Read the model definition and answer for the solid it produces. Units are mm, in the model's axes. Face numbers are marked on the shaded views. A direction names the side the tool comes from. Give positions to 0.01 mm unless a question says otherwise; leave off trailing zeros. Order: outer loops, then holes, each group sorted by start corner. A loop starts at its lowest first (then second) coordinate and runs counter-clockwise, first axis right, second up.
Item 1: The mould has two halves that part along Y. Classify the marked faces 3, 4 and 5: +Y half, -Y half, draft (parallel to the pull), parting line (faces both ways), or undercut.
Item 2: Given pin 1 Ø3 at (x, y) = (9, 6.5) entering from +Z; pin 2 Ø1.7 at (x, z) = (5, -26) entering from +Y; pin 3 Ø3 at (x, y) = (6, 4) entering from -Z, each flat-ended and moving along its own axis, determine where each tip first touches the part or whether it passes through.
Item 3: A cutting plane is placed at B-B (y = 5). Write down the section's boundary in (x, z), plus the area to 3 significant figures.
Item 4: A cutting plane is placed at A-A (z = -24). Write down the section's boundary in (x, y).
Item 5: A cutting plane is placed at C-C (x = 9). Write down the section's boundary in (y, z).
Item 6: Which of the six approach directions +Z, -Z, +X, -X, +Y, -Y give full straight-line access (tool end or side, diameter ignored) to the marked faces 1 and 2?
Item 7: Find the intervals of material crossed by line 1 along Z through (x, y) = (5, 0.55); line 2 along X through (y, z) = (0.9, -4); line 3 along Y through (x, z) = (5, -17.5), in increasing order.
from build123d import *

# Parameters (mm, degrees)
SKETCH1_R           = 4.5
BOSS_EXTRUDE1_DEPTH = 10
SKETCH2_R           = 1.9
CUT_EXTRUDE1_DEPTH  = 10
FILLET1_R           = 2
SKETCH3_R           = 1.9
CUT_EXTRUDE2_DEPTH  = 5


with BuildPart() as part:
    # Sketch1 → Boss-Extrude1 (new body)
    with BuildSketch(Plane(origin=(0, 0, 0), x_dir=(0, 0, -1), z_dir=(1, 0, 0))):
        with BuildLine():
            Line((0, 0), (28, 0))
            Line((28, 0), (28, 2))
            Line((28, 2), (19.766281297, 2))
            ThreePointArc((19.766281297, 2), (14, 11.5), (8.233718703, 2))
            Line((8.233718703, 2), (0, 2))
            Line((0, 2), (0, 0))
        make_face()
        with Locations((14, 5)):
            Circle(SKETCH1_R, mode=Mode.SUBTRACT)
    extrude(amount=BOSS_EXTRUDE1_DEPTH)

    # Sketch2 → Cut-Extrude1 (cut)
    with BuildSketch(Plane(origin=(0, 2, 0), x_dir=(1, 0, 0), z_dir=(0, 1, 0))):
        with Locations(Location((5, 24, 0), (0, 0, 270))):
            Circle(SKETCH2_R)
        with Locations(Location((5, 4, 0), (0, 0, 270))):
            Circle(SKETCH2_R)
    extrude(amount=-CUT_EXTRUDE1_DEPTH, mode=Mode.SUBTRACT)

    # Fillet1
    fillet1_edges = [part.edges().sort_by_distance(p)[0] for p in [
        (5, 2, -8.233718703),
        (5, 2, -19.766281297),
    ]]
    fillet(fillet1_edges, radius=FILLET1_R)

    # Sketch3 → Cut-Extrude2 (cut)
    with BuildSketch(Plane.XZ):
        with Locations(Location((5, -14, 0), (0, 0, 270))):
            Circle(SKETCH3_R)
    extrude(amount=-CUT_EXTRUDE2_DEPTH, mode=Mode.SUBTRACT)


solid = part.part
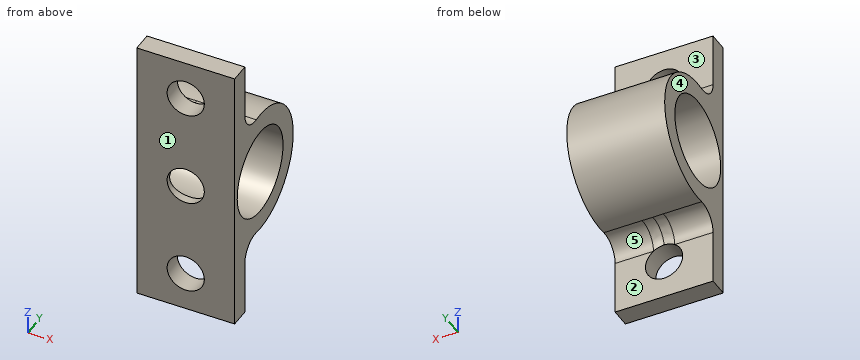
Response values:
1. face 3: +Y half
1. face 4: draft
1. face 5: undercut
2. pin 1: stops at z = -7.5
2. pin 2: stops at y = 2
2. pin 3: stops at z = -21.12
3. outline: (0, -20.5) - (10, -20.5) - (10, -18.5) - (0, -18.5) - close; (0, -9.5) - (10, -9.5) - (10, -7.5) - (0, -7.5) - close
3. area: 40.0 mm2
4. outline: (0, 0) - (3.1, 0) - (3.1, 2) - (0, 2) - close; (6.9, 0) - (10, 0) - (10, 2) - (6.9, 2) - close
5. outline: (0, -28) - (2, -28) - (2, -22.44) arc R2 cw to (4.24, -20.45) arc R6.5 ccw (long way) to (4.24, -7.55) arc R2 cw to (2, -5.56) - (2, 0) - (0, 0) - close; hole circle Ø9 at (5, -14)
6. face 1: +Z, -Z, +X, -X, -Y
6. face 2: -Z, +X, -X, +Y
7. line 1: z = -28 to -25.9, -22.1 to -15.9, -12.1 to -5.9, -2.1 to 0
7. line 2: x = 0 to 3.1, 6.9 to 10
7. line 3: y = 0 to 2.17, 7.83 to 10.48
